Model file for the job. Use its own axes, mm. Face numbers are marked on the shaded views. A direction names the side the tool comes from. Give positions to 0.01 mm unless a question says otherwise; leave off trailing zeros. Loops run counter-clockwise (first coordinate to the right, second up) from the corner with the lowest first, then second, coordinate; pieces in that order, holes last. Notation, with made-up numbers: M 68,23.25 L 103,23.25 A12 ccw 103,37.25 Z; hole C -7.5,40.5 d8. An arc over 180 degrees is marked long. Use CSV: the item, a comma, the result in double quotes. Start each with the question number.
(1) Tool access for the marked faces 1, 2, 3 and 4: list every direction of +Z, -Z, +X, -X, +Y, -Y with a clear straight run to the whole face (end or side of a thin tool).
(2) Slice it at D-D on y = -1.15. List the corners of the cut face in (x, z).
(3) Flat gauge pins, fed straight in: P1, Ø7.5, axis at x = 3.5, y = 2, coming from the +Z side; P2, Ø4, axis at y = -8, z = 9.5, coming from the -X side; P3, Ø1.2, axis at x = 25, y = -7.65, coming from the -Z side; P4, Ø5, axis at x = -2.5, y = -1, coming from the +Z side. Where does each tip first touch, or does it go through?
(4) Slice it at C-C on x = 25. List the corners of the cut face in (y, z).
(5) Slice it at A-A on z = 5.5. List the corners of the cut face in (x, y).
(6) Wall check: line 1 along Y through (x, z) = (25, 9.05); line 2 along Y through (x, z) = (25, 1.75); line 3 along Y through (x, z) = (16.5, 1.45). Give the ranges that are in metal, low to high. Write a range as from..to.
(7) Two-plate mould, pull along Y, no slides. Class the marked faces 5, 6, 7 and 8: pulls with the +Y half, pulls with the -Y half, needs draft (parallel to the pull), parting line crosses it, or undercut.
(8) Slice it at B-B on x = 16.5. List the corners of the cut face in (y, z), and give its area (3 significant figures).
```python
from build123d import *

# Parameters (mm, degrees)
F0_W     = 20
F0_H     = 23
F1_DEPTH = 5
F2_W     = 7
F2_H     = 3
F2_H_2   = 7.2
F2_R     = 1
F3_DEPTH = 5.8
F4_DEPTH = 5.001
F5_R     = 5
F6_R     = 1
F7_R     = 1
F8_DEPTH = 4
F2_R_2   = 1.5
F9_DEPTH = 5.001


with BuildPart() as f1:
    # F0 (on Top) → F1 (new body)
    with BuildSketch(Plane.XY):
        Rectangle(F0_W, F0_H)
        with BuildLine():
            Line((-3, 4.75), (3, 4.75))
            ThreePointArc((3, 4.75), (7.75, 0), (3, -4.75))
            Line((3, -4.75), (-3, -4.75))
            ThreePointArc((-3, -4.75), (-7.75, 0), (-3, 4.75))
        make_face(mode=Mode.SUBTRACT)
        with Locations((20, 0)):
            Rectangle(F0_W, F0_H)
    extrude(amount=F1_DEPTH)

    # F2 (on face) → F3 (join)
    with BuildSketch(Plane.XY.offset(5)):
        with Locations((26.5, 10)):
            Rectangle(F2_W, F2_H)
        with Locations((26.5, -7.9)):
            Rectangle(F2_W, F2_H_2)
        with Locations((25, -7.65)):
            Circle(F2_R, mode=Mode.SUBTRACT)
    extrude(amount=F3_DEPTH)

    # F2 (on face) → F4 (cut, through all)
    with BuildSketch(Plane.XY.offset(5)):
        with Locations((25, 5.35)):
            Circle(F2_R)
        with Locations((25, -1.15)):
            Circle(F2_R)
        with Locations((25, -7.65)):
            Circle(F2_R)
    extrude(amount=-F4_DEPTH, mode=Mode.SUBTRACT)

    # F5
    f5_edges = [f1.edges().sort_by_distance(p)[0] for p in [
        (-10, -11.5, 2.5),
        (-10, 11.5, 2.5),
    ]]
    fillet(f5_edges, radius=F5_R)

    # F6
    f6_edges = [f1.edges().sort_by_distance(p)[0] for p in [
        (30, -11.5, 5.4),
        (30, 11.5, 5.4),
    ]]
    fillet(f6_edges, radius=F6_R)

    # F7
    f7_edges = [f1.edges().sort_by_distance(p)[0] for p in [
        (23, 8.5, 7.9),
        (23, -4.3, 7.9),
        (30, -4.3, 7.9),
        (30, 8.5, 7.9),
        (23, -11.5, 7.9),
        (23, 11.5, 7.9),
    ]]
    fillet(f7_edges, radius=F7_R)

    # F0 (on Top) → F8 (join)
    with BuildSketch(Plane.XY):
        with BuildLine():
            ThreePointArc((3, -4.75), (7.75, 0), (3, 4.75))
            Line((3, 4.75), (-3, 4.75))
            ThreePointArc((-3, 4.75), (-7.75, 0), (-3, -4.75))
            Line((-3, -4.75), (3, -4.75))
        make_face()
        with BuildLine():
            Line((-3, 2.6), (3, 2.6))
            ThreePointArc((3, 2.6), (5.6, 0), (3, -2.6))
            Line((3, -2.6), (-3, -2.6))
            ThreePointArc((-3, -2.6), (-5.6, 0), (-3, 2.6))
        make_face(mode=Mode.SUBTRACT)
    extrude(amount=F8_DEPTH)

    # F2 (on face) → F9 (cut, through all)
    with BuildSketch(Plane.XY.offset(5)):
        with Locations((16.5, 1.5)):
            Circle(F2_R_2)
    extrude(amount=-F9_DEPTH, mode=Mode.SUBTRACT)


solid = f1.part
```
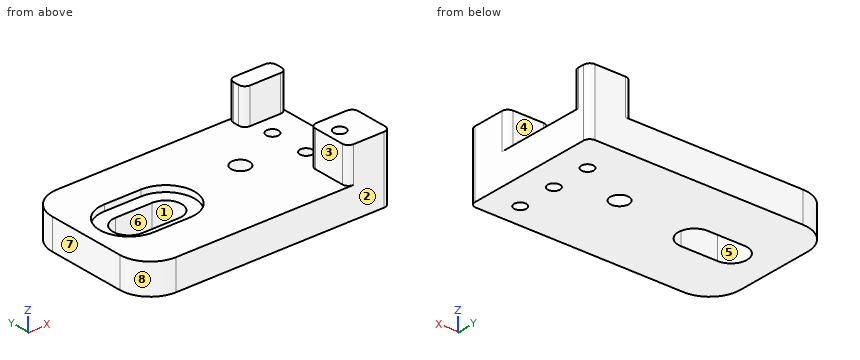
Reply:
1,face 1,"+Z, -Z"
1,face 2,"+Z, -Z, +X, -X, -Y"
1,face 3,"+Z, -X, +Y, -Y"
1,face 4,"+Z, +X, -X"
2,outline,"M -10,0 L -5.33,0 L -5.33,4 L -7.61,4 L -7.61,5 L -10,5 Z; M 5.33,0 L 24,0 L 24,5 L 7.61,5 L 7.61,4 L 5.33,4 Z; M 26,0 L 30,0 L 30,5 L 26,5 Z"
3,P1,"stops at z = 5"
3,P2,"stops at x = 23"
3,P3,"passes through"
3,P4,"stops at z = 4"
4,outline,"M -11.5,0 L -8.65,0 L -8.65,10.8 L -11.5,10.8 Z; M -6.65,0 L -2.15,0 L -2.15,5 L -4.3,5 L -4.3,10.8 L -6.65,10.8 Z; M -0.15,0 L 4.35,0 L 4.35,5 L -0.15,5 Z; M 6.35,0 L 11.5,0 L 11.5,10.8 L 8.5,10.8 L 8.5,5 L 6.35,5 Z"
5,outline,"M 23,-10.5 A1 ccw 24,-11.5 L 29,-11.5 A1 ccw 30,-10.5 L 30,-5.3 A1 ccw 29,-4.3 L 24,-4.3 A1 ccw 23,-5.3 Z; M 23,9.5 A1 ccw 24,8.5 L 29,8.5 A1 ccw 30,9.5 L 30,10.5 A1 ccw 29,11.5 L 24,11.5 A1 ccw 23,10.5 Z; hole C 25,-7.65 d2"
6,line 1,"y = -11.5..-8.65, -6.65..-4.3, 8.5..11.5"
6,line 2,"y = -11.5..-8.65, -6.65..-2.15, -0.15..4.35, 6.35..11.5"
6,line 3,"y = -11.5..0, 3..11.5"
7,face 5,"undercut"
7,face 6,"undercut"
7,face 7,"needs draft"
7,face 8,"pulls with the -Y half"
8,outline,"M -11.5,0 L 0,0 L 0,5 L -11.5,5 Z; M 3,0 L 11.5,0 L 11.5,5 L 3,5 Z"
8,area,"100 mm^2"
